Geometry: see drawing. Coordinates: mm, zero at the bounding-box minimum. A direction names the side the tool comes from. Give positions to 0.01 mm unless a question says otherwise; leave off trailing zeros. Loops run counter-clockwise (first coordinate to the right, second up) from the corner with the lowest first, then second, coordinate; pieces in that order, holes last. Notation, with made-up numbers: M 6.5,12 L 63.5,12 A18 ccw 63.5,31 Z; hole C 85,73.5 d6. An arc over 180 degrees is marked long. Put each result on its own line as item: value.
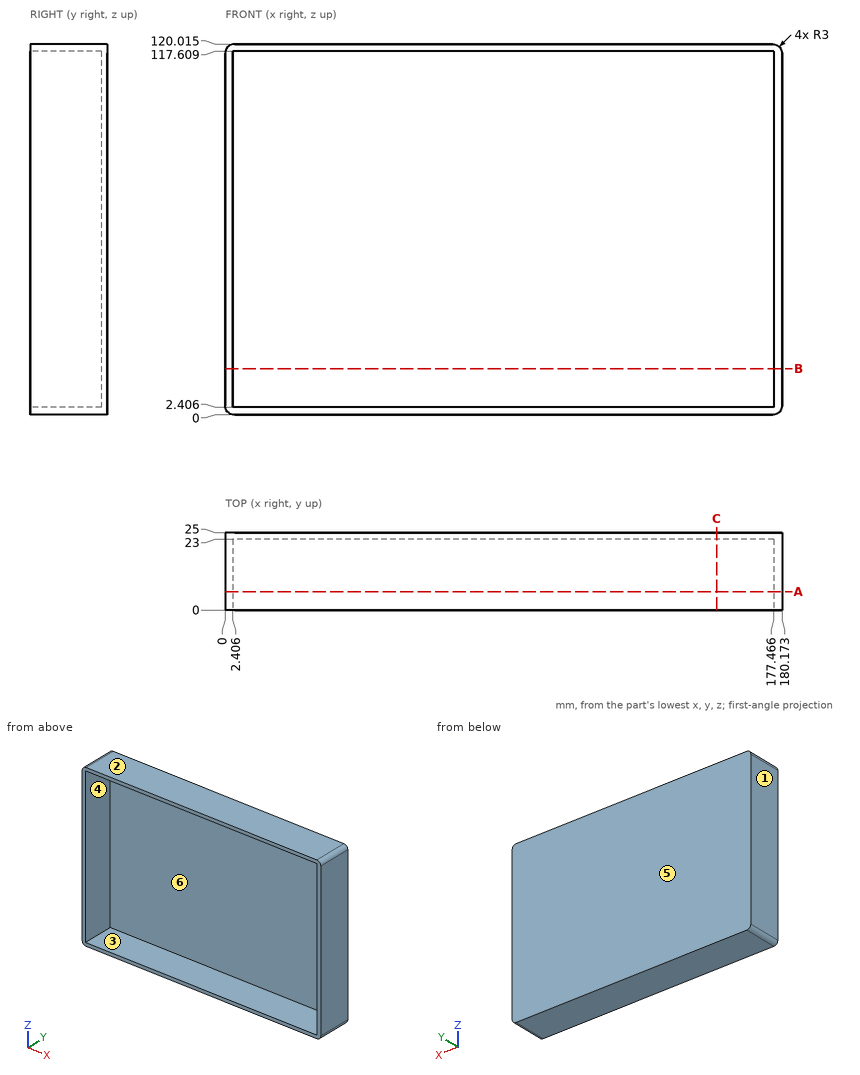
1. Section query C-C (x = 159). Output: boundary loops of the cut face in (y, z) (1 decimal).
Found:
outline: M 0,0 L 25,0 L 25,120 L 0,120 L 0,117.6 L 23,117.6 L 23,2.4 L 0,2.4 Z
2. Material intervals for line 1 (X direction, y = 2.5, z = 52); line 2 (Z direction, x = 157, y = 4.25) (1 decimal); line 3 (Y direction, x = 25.5, z = 67), sorted ascending. Write a range as from..to.
Found:
line 1: 0..2.41, 177.47..180.17
line 2: 0..2.4, 117.6..120
line 3: 23..25
3. Section query B-B (z = 15). Output: boundary loops of the cut face in (x, y).
Found:
outline: M 0,0 L 2.41,0 L 2.41,23 L 177.47,23 L 177.47,0 L 180.17,0 L 180.17,25 L 0,25 Z
4. Draft query along X for the marked faces 1, 2, 3 and 4. Return one class per face: pulls with the +X half, pulls with the -X half, needs draft (parallel to the pull), parting line crosses it, or undercut.
Found:
face 1: pulls with the -X half
face 2: needs draft
face 3: undercut
face 4: undercut
5. Section query A-A (y = 6). Output: boundary loops of the cut face in (x, z) (1 decimal).
Found:
outline: M 0,3 A3 ccw 3,0 L 177.2,0 A3 ccw 180.2,3 L 180.2,117 A3 ccw 177.2,120 L 3,120 A3 ccw 0,117 Z; hole M 2.4,2.4 L 177.5,2.4 L 177.5,117.6 L 2.4,117.6 Z
6. Access query for the marked faces 5 and 6. Directions: +Z, -Z, +X, -X, +Y, -Y. A direction counts if a zero-diameter tool reaches every point of the face in a straight line with its end or side. Return the directions, or none.
Found:
face 5: +Z, -Z, +X, -X, +Y
face 6: -Y
